Check sheet for the drawn part. Datum: minimum x, y, z corner. Units: mm. A direction names the side the tool comes from. Give positions to 0.01 mm unless a question says otherwise; leave off trailing zeros. Write each loop counter-clockwise with the first axis right and the second up, starting at its lowest first coordinate (ties: lowest second). Pieces come first, ordered by that corner, then holes. Notation, with made-up numbers: (28.5, 22.5) - (33.5, 22.5) arc R29 ccw to (33.5, 46.5) - close; hole circle Ø11 at (14.5, 81). An arc over 180 degrees is marked (long way). Answer as a JSON object with one key per item and string values. Group by question number.
Item 1: Sectioned sample at C-C, the plane x = 42.5. Record the boundary of the cut face in (y, z).
Item 2: Sectioned sample at D-D, the plane x = 30.5. Record the boundary of the cut face in (y, z), and give its area (3 significant figures).
Item 3: Sectioned sample at A-A, the plane z = 10. Record the boundary of the cut face in (x, y).
Item 4: Go/stop test with flat-tipped pins: pin 1 (1.6 mm diameter, centred on x = 34.5, y = 1, fed in from +Z); pin 2 (7 mm diameter, centred on x = 30.5, y = 63, fed in from +Z); pin 3 (0.7 mm diameter, centred on x = 36.5, y = 89.5, fed in from +Z). Record where each tip stops, or that it passes through.
Item 5: Draft check along Y on the marked faces 3, 4 and 5. Enter one of: +Y half, -Y half, draft (parallel to the pull), parting line (faces both ways), or undercut.
Item 6: Scan lines: line 1 along X through (y, z) = (39, 11.75); line 2 along Y through (x, z) = (23.5, 6.5); line 3 along Y through (x, z) = (34, 5.75) (1 decimal). Record each from-to range of solid material in increasing order. Write a range as [from, to].
Item 7: Sectioned sample at B-B, the plane y = 19. Record the boundary of the cut face in (x, z).
Item 8: Tool access check on the marked faces 1 and 2. Record the directions out of +Z, -Z, +X, -X, +Y, -Y that give a thin tool (end or side, any length) a straight path to the whole face; none if there is none.
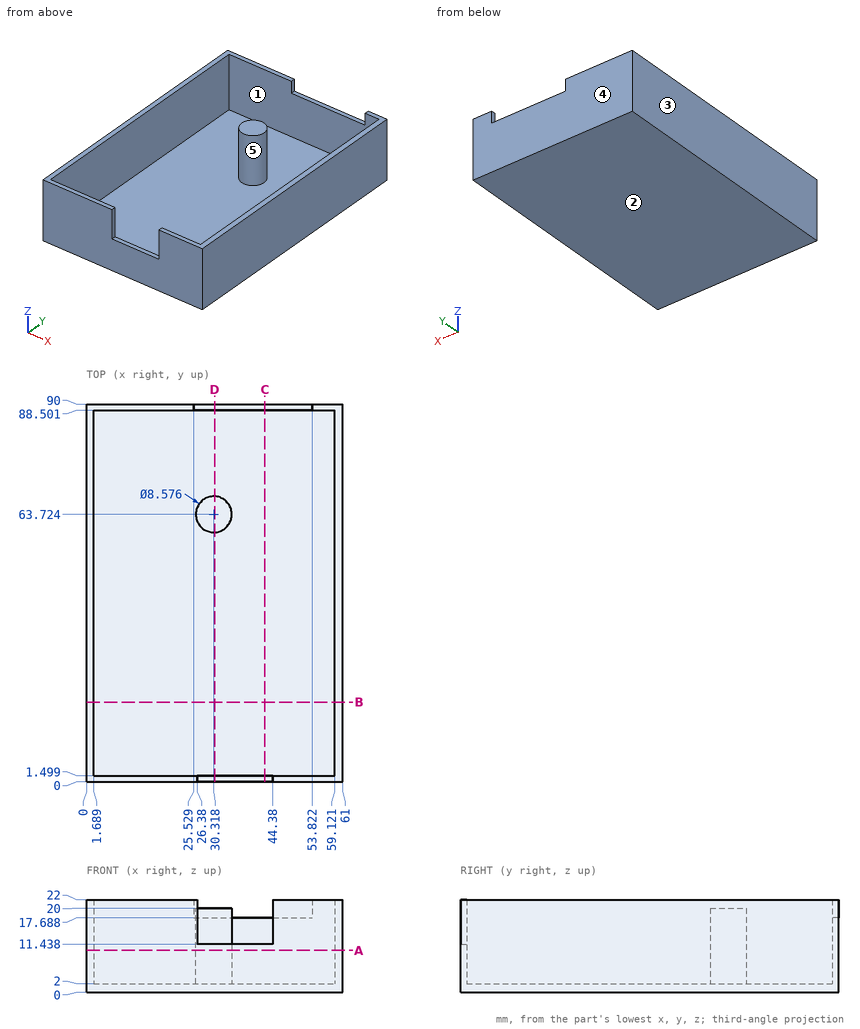
Geometry check:
{
 "1": {"outline": "(0, 0) - (90, 0) - (90, 17.69) - (88.5, 17.69) - (88.5, 2) - (1.5, 2) - (1.5, 11.44) - (0, 11.44) - close"},
 "2": {"outline": "(0, 0) - (90, 0) - (90, 17.69) - (88.5, 17.69) - (88.5, 2) - (68.01, 2) - (68.01, 20) - (59.44, 20) - (59.44, 2) - (1.5, 2) - (1.5, 11.44) - (0, 11.44) - close", "area": "372 mm^2"},
 "3": {"outline": "(0, 0) - (61, 0) - (61, 90) - (0, 90) - close; circle Ø8.58 at (30.32, 63.72); hole (1.69, 1.5) - (59.12, 1.5) - (59.12, 88.5) - (1.69, 88.5) - close"},
 "4": {"pin 1": "z = 11.44", "pin 2": "z = 20", "pin 3": "z = 17.69"},
 "5": {"face 3": "draft", "face 4": "+Y half", "face 5": "undercut"},
 "6": {"line 1": "[0, 1.69], [59.12, 61]", "line 2": "[0, 1.5], [88.5, 90]", "line 3": "[0, 1.5], [61.5, 65.9], [88.5, 90]"},
 "7": {"outline": "(0, 0) - (61, 0) - (61, 22) - (59.12, 22) - (59.12, 2) - (1.69, 2) - (1.69, 22) - (0, 22) - close"},
 "8": {"face 1": "+Z", "face 2": "-Z, +X, -X, +Y, -Y"}
}
